Build history of the part. All positions in model axes, mm. A direction names the side the tool comes from. Give positions to 0.01 mm unless a question says otherwise; leave off trailing zeros. Loops run counter-clockwise (first coordinate to the right, second up) from the corner with the lowest first, then second, coordinate; pieces in that order, holes last. Notation, with made-up numbers: (62, 45) -> (106, 45) arc R23 cw to (106, 77) -> close; hole circle Ø6 at (86.5, 9.25). An arc over 180 degrees is marked (long way). Answer in a Markdown table with one row per item. Add a question column.
from build123d import *

# Parameters (mm, degrees)
F3_D = 20


with BuildPart() as f1:
    # F0 (on Front) → F1 (revolve)
    with BuildSketch(Plane.XZ):
        Polygon((8, 38), (-8, 38), (-8, 3), (-12, 3), (-12, 0), (13, 0), (13, 6), (8, 6), align=None)
    revolve(axis=Axis((1.21409, 0, -13), (1, 0, 0)))

    # F3 (through all)
    with Locations(Plane.YZ.offset(8)):
        with Locations((0, 22), (-35, -13), (0, -48), (35, -13)):
            Hole(F3_D / 2)


solid = f1.part
(1) Flat gauge pins, fed straight in: pin 1 Ø8 at (x, y) = (-5.5, -0.5) entering from -Z; pin 2 Ø5 at (y, z) = (-3, 15) entering from +X; pin 3 Ø4 at (x, z) = (8, 20.5) entering from +Y; pin 4 Ø1.5 at (x, z) = (-4.5, 20) entering from -Y. Where does each tip first touch, or does it go through?
(2) Two-plate mould, pull along Z, no slides. Class faces 4 (the cylindrical face through (-10.03, 15.62, -16.47)), 5 (the cylindrical face through (-0.11, 2.17, -57.76)), 6 (the cylindrical face through (0, -27, -19)), 7 (the flat face through (8, -1, -35)): released by +Z, released by -Z, zero draft, split by the parting line, or undercut.
(3) Saw through at D-D, the plane y = 35. List the corners of the cut face in (x, z).
(4) 3-axis set-ups, long thin cutter, end or side, ignore diameter. For faces 1 (the cylindrical face through (0.7, -3.9, -0.6)), 2 (the flat face through (-8, -12, -2)), 3 (the cylindrical face through (10.465, 16.856, -4.233)): which of +Z, -Z, +X, -X, +Y, -Y reach the whole face in a straight line?
(5) Saw through at A-A, the plane y = 0. List the corners of the cut face in (x, z), then the cut area to 3 significant figures.
(6) Saw through at B-B, the plane z = -13. List the corners of the cut face in (x, y).
(7) Saw through at C-C, the plane x = -5.75. List the corners of the cut face in (y, z).
(8) Wall check: line 1 along Z through (x, y) = (-4.5, 0); line 2 along Z through (x, y) = (3.5, 3); line 3 along X through (y, z) = (-21, -51). Give the ranges that are in metal, low to high. Write a range as from..to.
Worked answers:
| question | item | result |
|---|---|---|
| 1 | pin 1 | z = -64 |
| 1 | pin 2 | x = 8 |
| 1 | pin 3 | y = 40.11 |
| 1 | pin 4 | y = -39.51 |
| 2 | face 4 | split by the parting line |
| 2 | face 5 | undercut |
| 2 | face 6 | undercut |
| 2 | face 7 | zero draft |
| 3 | outline | (-8, -50.09) -> (8, -50.09) -> (8, -23) -> (-8, -23) -> close; (-8, -3) -> (8, -3) -> (8, 24.09) -> (-8, 24.09) -> close |
| 4 | face 1 | +X, -X |
| 4 | face 2 | -X |
| 4 | face 3 | +X |
| 5 | outline | (-12, -29) -> (-8, -29) -> (-8, -38) -> (8, -38) -> (8, -32) -> (13, -32) -> (13, -26) -> (-12, -26) -> close; (-12, 0) -> (13, 0) -> (13, 6) -> (8, 6) -> (8, 12) -> (-8, 12) -> (-8, 3) -> (-12, 3) -> close; (-8, -64) -> (8, -64) -> (8, -58) -> (-8, -58) -> close; (-8, 32) -> (8, 32) -> (8, 38) -> (-8, 38) -> close |
| 5 | area | 660 mm^2 |
| 6 | outline | (-12, -16) -> (-8, -16) -> (-8, -25) -> (8, -25) -> (8, -19) -> (13, -19) -> (13, -13) -> (-12, -13) -> close; (-12, 13) -> (13, 13) -> (13, 19) -> (8, 19) -> (8, 25) -> (-8, 25) -> (-8, 16) -> (-12, 16) -> close; (-8, -51) -> (8, -51) -> (8, -45) -> (-8, -45) -> close; (-8, 45) -> (8, 45) -> (8, 51) -> (-8, 51) -> close |
| 7 | outline | circle Ø102 at (0, -13); hole circle Ø20 at (-35, -13); hole circle Ø26 at (0, -13); hole circle Ø20 at (0, -48); hole circle Ø20 at (0, 22); hole circle Ø20 at (35, -13) |
| 8 | line 1 | -64..-58, -38..-26, 0..12, 32..38 |
| 8 | line 2 | -63.91..-57.54, -38.46..-25.65, -0.35..12.46, 31.54..37.91 |
| 8 | line 3 | -8..8 |
